from build123d import *

# Parameters (mm, degrees)
F2_DEPTH = 76.2
F3_R     = 12.538791
F4_DEPTH = 54.609487
F6_DEPTH = 12.7


with BuildPart() as f2:
    # F0 (on Front) → F2 (new body)
    with BuildSketch(Plane.XZ):
        Polygon((-54.608487, 0), (0, 0), (-28.783787, 44.618372), (-54.608487, 44.618372), align=None)
    extrude(amount=F2_DEPTH)

    # F3 (on face) → F4 (cut, through all)
    with BuildSketch(Plane(origin=(-54.608487, 0, 0), x_dir=(0, -1, 0), z_dir=(-1, 0, 0))):
        with Locations((33.949289, 21.771144)):
            Circle(F3_R)
    extrude(amount=-F4_DEPTH, mode=Mode.SUBTRACT)

    # F5 (on Front) → F6 (join)
    with BuildSketch(Plane.XZ):
        Polygon((-54.608487, 54.538789), (-54.608487, 44.618372), (-28.783787, 44.618372), (0, 0), (9.920417, 0), (-25.263137, 54.538789), align=None)
    extrude(amount=F6_DEPTH)


solid = f2.part
Input: part model. Units: mm. Frame: model coordinates. A direction names the side the tool comes from. Round coordinates to 2 decimals unless told otherwise and drop trailing zeros. Write each loop counter-clockwise with the first axis right and the second up, starting at its lowest first coordinate (ties: lowest second). Pieces come first, ordered by that corner, then holes.
1) Cut plane B-B (x = -41). Return the cut outline in (y, z).
2) Cut plane A-A (z = 26.5). Return the cut outline in (x, y).
3) Reachability of faces 1 (the flat face through (-7.425, -6.261, 26.888)), 2 (the flat face through (-42, -44, 44.618)) from +Z, -Z, +X, -X, +Y, -Y: full face, straight path, thin tool, end or side. Return the list, or none.
4) Ray query, L1, parallel to Y at x = -11, z = 20; L2, parallel to Y at x = -25, z = 29; L3, parallel to Z at x = -43, y = -54. Return the intervals inside material, ascending.
5) Draft query along Y for faces 3 (the cylindrical face through (-35.95, -31.23, 9.53)), 4 (the flat face through (-14.19, -51.061, 21.997)), 5 (the flat face through (-22, -12.7, 35)). Return one class per face: pulls with the +Y half, pulls with the -Y half, needs draft (parallel to the pull), parting line crosses it, or undercut.
6) Cut plane D-D (y = -50). Return the cut outline in (x, z).
7) Contact query for flat-ended pins moving along their axis: P1, Ø12, axis at x = -14, z = 35, coming from the -Y side; P2, Ø7.5, axis at x = -37.5, y = -56.5, coming from the +Z side; P3, Ø12, axis at y = -18, z = 13, coming from the +X side. Output: stop coordinate, or through.
8) Cut plane C-C (x = -18). Return the cut outline in (y, z), then the cut area to 3 significant figures.
Geometry says:
1. outline: (-76.2, 0) - (0, 0) - (0, 54.54) - (-12.7, 54.54) - (-12.7, 44.62) - (-76.2, 44.62) - close; hole circle Ø25.08 at (-33.95, 21.77)
2. outline: (-54.61, -76.2) - (-17.1, -76.2) - (-17.1, -45.56) - (-54.61, -45.56) - close; (-54.61, -22.34) - (-17.1, -22.34) - (-17.1, -12.7) - (-7.18, -12.7) - (-7.18, 0) - (-54.61, 0) - close
3. face 1: +Z, +X, +Y, -Y
3. face 2: +Z, +X, -X, -Y
4. L1: y = -12.7 to 0
4. L2: y = -76.2 to -44.19, -23.7 to 0
4. L3: z = 0 to 44.62
5. face 3: undercut
5. face 4: needs draft
5. face 5: pulls with the -Y half
6. outline: (-54.61, 0) - (0, 0) - (-28.78, 44.62) - (-54.61, 44.62) - close
7. P1: stops at y = -12.7
7. P2: stops at z = 44.62
7. P3: stops at x = 3.35
8. outline: (-76.2, 0) - (0, 0) - (0, 43.28) - (-12.7, 43.28) - (-12.7, 27.9) - (-23.01, 27.9) arc R12.54 cw (long way) to (-44.89, 27.9) - (-76.2, 27.9) - close
8. area: 1,930 mm2
